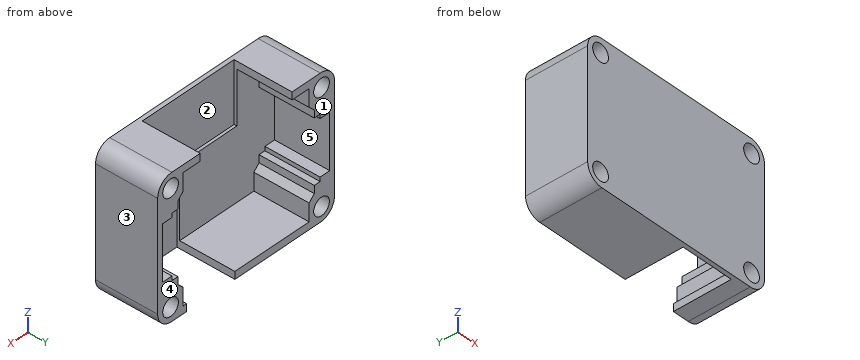
```python
from build123d import *

# Parameters (mm, degrees)
BOSS_EXTRUDE1_DEPTH = 16
BOSS_EXTRUDE2_DEPTH = 2
SKETCH3_W           = 15.3
SKETCH3_H           = 16.8
CUT_EXTRUDE1_DEPTH  = 16.8
SKETCH4_R           = 2.5
CUT_EXTRUDE2_DEPTH  = 19
SKETCH5_W           = 29.15
SKETCH5_H           = 16.8
CUT_EXTRUDE3_DEPTH  = 17.5


with BuildPart() as part:
    # Sketch1 → Boss-Extrude1 (new body)
    with BuildSketch(Plane(origin=(0, 0, 0), x_dir=(1, 0, 0), z_dir=(0, 1, 0))):
        with BuildLine():
            Line((23.55, 20.15), (-23.55, 20.15))
            ThreePointArc((-23.55, 20.15), (-26.731980515, 18.831980515), (-28.05, 15.65))
            Line((-28.05, 15.65), (-28.05, -15.65))
            ThreePointArc((-28.05, -15.65), (-26.731980515, -18.831980515), (-23.55, -20.15))
            Line((-23.55, -20.15), (23.55, -20.15))
            ThreePointArc((23.55, -20.15), (26.731980515, -18.831980515), (28.05, -15.65))
            Line((28.05, -15.65), (28.05, 15.65))
            ThreePointArc((28.05, 15.65), (26.731980515, 18.831980515), (23.55, 20.15))
        make_face()
        Polygon((-20, -18), (20, -18), (20, -12.9), (21.65, -11.3), (21.65, -9.1), (23.5, -9.1), (23.5, -7.9), (26.55, -7.9), (26.55, 7.9), (23.5, 7.9), (23.5, 9.1), (21.65, 9.1), (21.65, 11.3), (20, 12.9), (20, 18), (-20, 18), (-20, 12.9), (-21.65, 11.3), (-21.65, 9.1), (-23.5, 9.1), (-23.5, 7.9), (-26.55, 7.9), (-26.55, -7.9), (-23.5, -7.9), (-23.5, -9.1), (-21.65, -9.1), (-21.65, -11.3), (-20, -12.9), align=None, mode=Mode.SUBTRACT)
    extrude(amount=BOSS_EXTRUDE1_DEPTH)

    # Sketch2 → Boss-Extrude2 (add)
    with BuildSketch(Plane.XZ):
        with BuildLine():
            Line((-23.55, -20.15), (23.55, -20.15))
            ThreePointArc((23.55, -20.15), (26.731980515, -18.831980515), (28.05, -15.65))
            Line((28.05, -15.65), (28.05, 15.65))
            ThreePointArc((28.05, 15.65), (26.731980515, 18.831980515), (23.55, 20.15))
            Line((23.55, 20.15), (-23.55, 20.15))
            ThreePointArc((-23.55, 20.15), (-26.731980515, 18.831980515), (-28.05, 15.65))
            Line((-28.05, 15.65), (-28.05, -15.65))
            ThreePointArc((-28.05, -15.65), (-26.731980515, -18.831980515), (-23.55, -20.15))
        make_face()
    extrude(amount=BOSS_EXTRUDE2_DEPTH)

    # Sketch3 → Cut-Extrude1 (cut)
    with BuildSketch(Plane(origin=(0, 0, -20.15), x_dir=(-1, 0, 0), z_dir=(0, 0, -1))):
        with Locations((-11.2, 7.6)):
            Rectangle(SKETCH3_W, SKETCH3_H)
    extrude(amount=-CUT_EXTRUDE1_DEPTH, mode=Mode.SUBTRACT)

    # Sketch4 → Cut-Extrude2 (cut, through all)
    with BuildSketch(Plane(origin=(0, 16, 0), x_dir=(1, 0, 0), z_dir=(0, 1, 0))):
        with Locations((23.95, 16.069558847)):
            Circle(SKETCH4_R)
        with Locations((23.95, -16.069558847)):
            Circle(SKETCH4_R)
        with Locations((-23.95, 16.069558847)):
            Circle(SKETCH4_R)
        with Locations((-23.95, -16.069558847)):
            Circle(SKETCH4_R)
    extrude(amount=-CUT_EXTRUDE2_DEPTH, mode=Mode.SUBTRACT)

    # Sketch5 → Cut-Extrude3 (cut)
    with BuildSketch(Plane.XY.offset(20.15)):
        with Locations((-0.025, 7.6)):
            Rectangle(SKETCH5_W, SKETCH5_H)
    extrude(amount=-CUT_EXTRUDE3_DEPTH, mode=Mode.SUBTRACT)


solid = part.part
```
Can you work these out from the model? Positions are in its coordinate system, mm. Face numbers are marked on the shaded views. A direction names the side the tool comes from. Round coordinates to 2 decimals unless told otherwise and drop trailing zeros. Order: outer loops, then holes, each group sorted by start corner. A loop starts at its lowest first (then second) coordinate and runs counter-clockwise, first axis right, second up.
(1) If I drill on L1, parallel to X at y = 1, z = -16; L2, parallel to X at y = 11.25, z = -4.5; L3, parallel to X at y = 12.5, z = -10.5, over which ranges is the centre line in solid material (lowest first)?
Results are:
L1: x = -28.04 to -26.45, -21.45 to -20, 20 to 21.45, 26.45 to 28.04
L2: x = -28.05 to -26.55, 26.55 to 28.05
L3: x = -28.05 to -21.65, 21.65 to 28.05
(2) On a 3-axis mill with a long thin cutter (end or side, diameter ignored), from which of +Z, -Z, +X, -X, +Y, -Y can I reach the whole of each face in a straight line? I mean the marked faces 4 and 5. Say none if no direction works.
Results are:
face 4: +Z, -Z, +X, -X, +Y
face 5: +Y
(3) I'm going to push flat-ended pins straight in: pin 1 (4 mm diameter, centred on x = 6, y = 4.5, fed in from -Z) (3 decimals); pin 2 (8 mm diameter, centred on x = -10.5, y = 9.5, fed in from +Z); pin 3 (1.5 mm diameter, centred on x = -25, y = 4, fed in from -Z). Where does each tip first touch, or does it pass through?
Results are:
pin 1: passes through
pin 2: stops at z = -18
pin 3: stops at z = -20.1
(4) If we section it at D-D (z = -17): Please give me the cut outline in (x, y), plus the area to 3 significant figures.
Results are:
outline: (-27.84, -2) - (-26.27, -2) - (-26.27, 16) - (-27.84, 16) - close; (-21.63, -2) - (21.63, -2) - (21.63, 16) - (20, 16) - (20, 0) - (18.85, 0) - (18.85, -0.8) - (3.55, -0.8) - (3.55, 0) - (-20, 0) - (-20, 16) - (-21.63, 16) - close; (26.27, -2) - (27.84, -2) - (27.84, 16) - (26.27, 16) - close
area: 183 mm2
(5) If we section it at A-A (x = 0): Please give me the cut outline in (y, z), plus the area to 3 significant figures.
Results are:
outline: (-2, -20.15) - (16, -20.15) - (16, -18) - (0, -18) - (0, 2.65) - (-0.8, 2.65) - (-0.8, 20.15) - (-2, 20.15) - close
area: 101 mm2
(6) If we section it at B-B (z = -2): Please give me the cut outline in (x, y), plus the area to 3 significant figures.
Results are:
outline: (-28.05, -2) - (28.05, -2) - (28.05, 16) - (26.55, 16) - (26.55, 0) - (-26.55, 0) - (-26.55, 16) - (-28.05, 16) - close
area: 160 mm2
(7) If we section it at C-C (y = 4): Count the separate pieces of the cut face and the enclosed holes in it, plus the area to 3 significant figures.
Results are:
separate pieces: 2
enclosed holes: 4
area: 386 mm2
(8) We'd pull the mould along X, two halves only. Please class the marked faces 1, 2 and 3: +X half, -X half, draft (parallel to the pull), parting line (faces both ways), or undercut.
Results are:
face 1: draft
face 2: undercut
face 3: +X half
